Verification items for the finished model (mm, model axes). Face numbers are marked on the shaded views. Give positions to 0.01 mm unless a question says otherwise; leave off trailing zeros. Loops run counter-clockwise (first coordinate to the right, second up) from the corner with the lowest first, then second, coordinate; pieces in that order, holes last. Notation, with made-up numbers: M 44.5,-7 L 84.5,-7 A23 cw 84.5,12 Z; hole C 73,42 d8. An arc over 180 degrees is marked long. Answer in a Markdown table with one row per item.
```python
from build123d import *

# Parameters (mm, degrees)
SKETCH2_R           = 101.6
SKETCH2_R_2         = 95.25
BOSS_EXTRUDE1_DEPTH = 374.65
SKETCH3_W           = 31.75
SKETCH3_H           = 50.8
CUT_EXTRUDE2_DEPTH  = 402.257700861
SKETCH4_R           = 2.5
CUT_EXTRUDE3_DEPTH  = 402.257700861


with BuildPart() as part:
    # Sketch2 → Boss-Extrude1 (new body)
    with BuildSketch(Plane(origin=(0, 0, 0), x_dir=(1, 0, 0), z_dir=(0, 1, 0))):
        with Locations(Location((0, 0, 0), (0, 0, 90))):
            Circle(SKETCH2_R)
        with Locations(Location((0, 0, 0), (0, 0, 90))):
            Circle(SKETCH2_R_2, mode=Mode.SUBTRACT)
    extrude(amount=BOSS_EXTRUDE1_DEPTH)

    # Sketch3 → Cut-Extrude2 (cut, through all)
    with BuildSketch(Plane.XY):
        with Locations((-85.725, 323.886005252)):
            Rectangle(SKETCH3_W, SKETCH3_H)
    extrude(amount=-CUT_EXTRUDE2_DEPTH, mode=Mode.SUBTRACT)

    # Sketch4 → Cut-Extrude3 (cut, through all)
    with BuildSketch(Plane(origin=(0, 0, 0), x_dir=(0, 0, -1), z_dir=(1, 0, 0))):
        with Locations((81.400332745, 356.906005252)):
            Circle(SKETCH4_R)
        with Locations((36.890166373, 356.906005252)):
            Circle(SKETCH4_R)
        with Locations((-7.62, 356.906005252)):
            Circle(SKETCH4_R)
        with Locations((-7.62, 323.886005252)):
            Circle(SKETCH4_R)
        with Locations((-7.62, 290.866005252)):
            Circle(SKETCH4_R)
        with Locations((36.890166373, 290.866005252)):
            Circle(SKETCH4_R)
        with Locations((81.400332745, 290.866005252)):
            Circle(SKETCH4_R)
        with Locations((81.400332745, 323.886005252)):
            Circle(SKETCH4_R)
    extrude(amount=-CUT_EXTRUDE3_DEPTH, mode=Mode.SUBTRACT)


solid = part.part
```
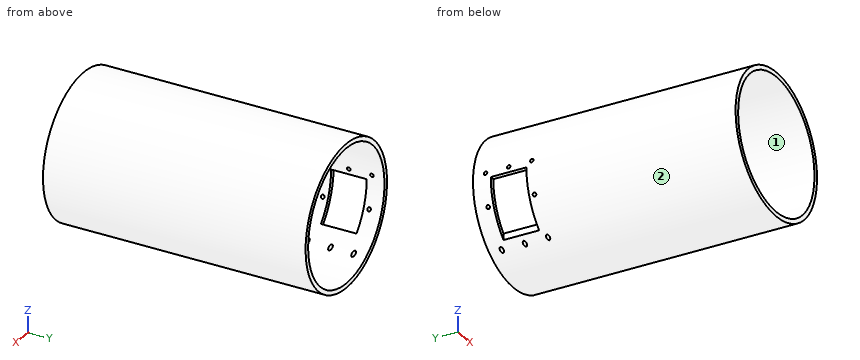
Item 1: Sectioned sample at B-B (z = 68). Record the cut outline in (x, y).
Reported:
| item | result |
|---|---|
| outline | M -75.49,0 L -66.7,0 L -66.7,374.65 L -75.49,374.65 Z; M 66.7,0 L 75.49,0 L 75.49,374.65 L 66.7,374.65 Z |
Item 2: Go/stop test with flat-tipped pins: pin 1 (4 mm diameter, centred on y = 282, z = 65.5, fed in from -X); pin 2 (8 mm diameter, centred on y = 290.87, z = -81.4, fed in from -X); pin 3 (4.5 mm diameter, centred on y = 290.87, z = 7.62, fed in from -X). Record where each tip stops, or that it passes through.
Reported:
| item | result |
|---|---|
| pin 1 | stops at x = -79.31 |
| pin 2 | stops at x = -65.82 |
| pin 3 | stops at x = 94.74 |
Item 3: Sectioned sample at C-C (x = -76). Record the cut outline in (y, z).
Reported:
| item | result |
|---|---|
| outline | M 0,-67.43 L 298.49,-67.43 L 298.49,-57.42 L 0,-57.42 Z; M 0,57.42 L 374.65,57.42 L 374.65,67.43 L 0,67.43 Z; M 349.29,-67.43 L 374.65,-67.43 L 374.65,-57.42 L 349.29,-57.42 Z |
Item 4: Scan lines: L1, parallel to Y at x = -97, z = 7.62; L2, parallel to X at y = 68, z = -3; L3, parallel to Z at x = -53, y = 204.5. Record each from-to range of solid material in increasing order. Write a range as [from, to].
Reported:
| item | result |
|---|---|
| L1 | y = [0, 288.37], [293.37, 321.39], [326.39, 354.41], [359.41, 374.65] |
| L2 | x = [-101.56, -95.2], [95.2, 101.56] |
| L3 | z = [-86.68, -79.14], [79.14, 86.68] |
Item 5: Sectioned sample at D-D (z = -57). Record the cut outline in (x, y), and give its area (3 significant figures).
Reported:
| item | result |
|---|---|
| outline | M -84.1,0 L -76.31,0 L -76.31,298.49 L -84.1,298.49 Z; M -84.1,349.29 L -76.31,349.29 L -76.31,374.65 L -84.1,374.65 Z; M 76.31,0 L 84.1,0 L 84.1,374.65 L 76.31,374.65 Z |
| area | 5,440 mm^2 |
Item 6: Release check for a two-part mould opening along Z. For the marked faces 1 and 2 record: released by +Z, released by -Z, zero draft, split by the parting line, or undercut.
Reported:
| item | result |
|---|---|
| face 1 | undercut |
| face 2 | split by the parting line |
Item 7: Sectioned sample at A-A (x = 0). Record the cut outline in (y, z).
Reported:
| item | result |
|---|---|
| outline | M 0,-101.6 L 374.65,-101.6 L 374.65,-95.25 L 0,-95.25 Z; M 0,95.25 L 374.65,95.25 L 374.65,101.6 L 0,101.6 Z |
